from build123d import *

# Parameters (mm, degrees)
F0_R     = 65
F0_R_2   = 4
F1_DEPTH = 30
F2_R     = 15
F4_DEPTH = 50
F5_R     = 1.9999


# Not quite as in the source:
# - a fillet or chamfer is up to 0.001 mm smaller than in the source, because OpenCascade refuses the exact size


with BuildPart() as f1:
    # F0 (on Top) → F1 (new body, symmetric)
    with BuildSketch(Plane.XY):
        Circle(F0_R)
        Circle(F0_R_2, mode=Mode.SUBTRACT)
    extrude(amount=F1_DEPTH, both=True)

    # F2
    f2_edges = [f1.edges().sort_by_distance(p)[0] for p in [
        (-4, 0, 30),
        (4, 0, 0),
        (-4, 0, -30),
        (-65, 0, -30),
        (65, 0, 0),
        (-65, 0, 30),
    ]]
    fillet(f2_edges, radius=F2_R)

    # F3 (on Top) → F4 (join)
    with BuildSketch(Plane.XY):
        with BuildLine():
            Line((2.5, -62.9519052838), (-2.5, -62.9519052838))
            ThreePointArc((-2.5, -62.9519052838), (-4.5, -64.9519052838), (-2.5, -66.9519052838))
            Line((-2.5, -66.9519052838), (2.5, -66.9519052838))
            ThreePointArc((2.5, -66.9519052838), (4.5, -64.9519052838), (2.5, -62.9519052838))
        make_face()
    extrude(amount=F4_DEPTH)

    # F5 (radius 2 in the source; OpenCascade refuses exactly that, so slightly less here)
    f5_edges = [f1.edges().sort_by_distance(p)[0] for p in [
        (0, -66.951905, 0),
    ]]
    fillet(f5_edges, radius=F5_R)


solid = f1.part
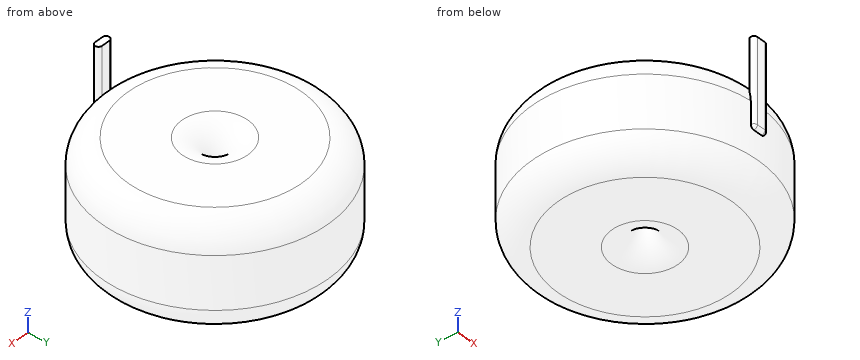
Input: part model. Units: mm. Frame: model coordinates. Round coordinates to 2 decimals unless told otherwise and drop trailing zeros. Write each loop counter-clockwise with the first axis right and the second up, starting at its lowest first coordinate (ties: lowest second). Pieces come first, ordered by that corner, then holes.
1) Contact query for flat-ended pins moving along their axis: P1, Ø12, axis at y = 3.5, z = 41.5, coming from the -X side; P2, Ø8, axis at y = 14.5, z = 7.5, coming from the -X side; P3, Ø1, axis at x = 43, y = 17, coming from the +Z side; P4, Ø5.5, axis at x = 1, z = 38.5, coming from the +Y side. Output: stop coordinate, or through.
2) Cut plane C-C (z = 38.5). Return the cut outline in (x, y).
3) Cut plane B-B (z = -7). Return the cut outline in (x, y).
4) Cut plane D-D (z = 8.5). Return the cut outline in (x, y), then the cut area to 3 significant figures.
5) Cut plane A-A (y = 0). Return the cut outline in (x, z).
6) Ray query, L1, parallel to Y at x = 0, z = -9; L2, parallel to Y at x = 0, z = 4.5; L3, parallel to Z at x = -41.5, y = 19.5. Return the intervals inside material, ascending.
Geometry says:
1. P1: passes through
1. P2: stops at x = -64.15
1. P3: stops at z = 30
1. P4: stops at y = -62.95
2. outline: (-2.5, -66.95) - (2.5, -66.95) arc R2 ccw to (2.5, -62.95) - (-2.5, -62.95) arc R2 ccw to start
3. outline: circle Ø130 at (0, 0); hole circle Ø8 at (0, 0)
4. outline: (-4.5, -64.84) arc R2 ccw to (-2.5, -66.95) - (2.5, -66.95) arc R2 ccw to (4.5, -64.84) arc R65 ccw (long way) to start; hole circle Ø8 at (0, 0)
4. area: 13,200 mm2
5. outline: (-65, -15) arc R15 ccw to (-50, -30) - (-19, -30) arc R15 ccw to (-4, -15) - (-4, 15) arc R15 ccw to (-19, 30) - (-50, 30) arc R15 ccw to (-65, 15) - close; (4, -15) arc R15 ccw to (19, -30) - (50, -30) arc R15 ccw to (65, -15) - (65, 15) arc R15 ccw to (50, 30) - (19, 30) arc R15 ccw to (4, 15) - close
6. L1: y = -65 to -4, 4 to 65
6. L2: y = -66.95 to -4, 4 to 65
6. L3: z = -30 to 30
